Verification items for the finished model (mm, model axes). A direction names the side the tool comes from. Coordinates: 2 decimals unless noted, no trailing zeros. Order: outer loops, then holes, each group sorted by start corner. A loop starts at its lowest first (then second) coordinate and runs counter-clockwise, first axis right, second up. Notation, with made-up numbers: (16, 58) -> (64, 58) arc R7 cw to (64, 67) -> close; hole circle Ø7 at (-12, 79.5). An arc over 180 degrees is marked (long way). Write each question's results on one line, items separated by ' | '. Start each with the question number.
(1) Set-up check for faces 1 (the cylindrical face through (8.767, -16.856, 24.363)), 2 (the flat face through (-15.92, 38.95, 6.9)), 3 (the flat face through (-38.95, -15.92, 6.9)): record each of +Z, -Z, +X, -X, +Y, -Y from which the full face is reachable in a straight line by a thin tool's end or side.
(2) Cross-section at A-A on y = 2. Enter the section's corners in (x, z).
(3) Cross-section at B-B on z = 19.75. Enter the section's corners in (x, y), and give its area (3 significant figures).
(4) Cross-section at C-C on y = -14. Enter the section's corners in (x, z), and give its area (3 significant figures).
(5) Cross-section at D-D on y = 17.5. Enter the section's corners in (x, z).
(6) Draft check along Y on faces 4 (the flat face through (-41.078, -11.007, 6.902)), 5 (the flat face through (-25.46, 33.5, 6.9)), 6 (the flat face through (25.46, -33.5, 6.9)), 7 (the flat face through (-14, 27, 0)). Enter one of: +Y half, -Y half, draft (parallel to the pull), parting line (faces both ways), or undercut.
(7) Thickness scan on probe 1 along Y at (x, z) = (0, 21); probe 2 along Z at (x, y) = (36, 4.5); probe 3 along Y at (x, z) = (15, 23.75). Record the ranges inside material, lowest first. Write a range as [from, to].
(8) Go/stop test with flat-tipped pins: pin 1 (0.8 mm diameter, centred on y = 12, z = 13.5, fed in from -X); pin 2 (5 mm diameter, centred on y = 22, z = 14, fed in from +X); pin 3 (10 mm diameter, centred on x = 31.5, z = 14.5, fed in from -Y). Record where each tip stops, or that it passes through.
```python
from build123d import *

# Parameters (mm, degrees)
SKETCH1_R                  = 45
BOSS_EXTRUDE1_DEPTH        = 14
SKETCH2_R                  = 20
BOSS_EXTRUDE2_DEPTH        = 14
CUT_EXTRUDE1_DEPTH         = 70.526973183
CUT_EXTRUDE1_DEPTH_BACK    = 70.526973183
SKETCH3_R                  = 11
CUT_EXTRUDE2_DEPTH         = 70.526973183
CUT_EXTRUDE2_DEPTH_BACK    = 6
SKETCH4_R                  = 30
CUT_EXTRUDE3_DEPTH         = 70.526973183
CUT_EXTRUDE3_DEPTH_BACK    = 70.526973183
SKETCH5_W                  = 6
SKETCH5_H                  = 4.8
CUT_EXTRUDE4_DEPTH         = 70.526973183
FILLET1_R                  = 0.4
CIRPATTERN1_DEPTH          = 14
CUT_J8_CIRCLIPGROOVE_START = 23.5
SKETCH_J8_GROOVE_R         = 21.5
SKETCH_J8_GROOVE_R_2       = 19
CUT_J8_CIRCLIPGROOVE_DEPTH = 1.75


# Read off the part's stored shape, not the designer's step: CirPattern1
with BuildPart() as part:
    # Sketch1 → Boss-Extrude1 (new body)
    with BuildSketch(Plane.XY):
        Circle(SKETCH1_R)
    extrude(amount=BOSS_EXTRUDE1_DEPTH)

    # Sketch2 → Boss-Extrude2 (add)
    with BuildSketch(Plane.XY.offset(14)):
        Circle(SKETCH2_R)
    extrude(amount=BOSS_EXTRUDE2_DEPTH)

    # Sketch3 → Cut-Extrude1 (cut, two sides: drawn at the far end of the back side and taken through both)
    with BuildSketch(Plane.XY.offset(28).offset(-CUT_EXTRUDE1_DEPTH_BACK)):
        Circle(SKETCH3_R)
    extrude(amount=CUT_EXTRUDE1_DEPTH + CUT_EXTRUDE1_DEPTH_BACK, mode=Mode.SUBTRACT)

    # Sketch4 → Cut-Extrude2 (cut, two sides: drawn at the far end of the back side and taken through both)
    with BuildSketch(Plane(origin=(0, 0, 0), x_dir=(-1, 0, 0), z_dir=(0, 0, -1)).offset(-CUT_EXTRUDE2_DEPTH_BACK)):
        Circle(SKETCH4_R)
    extrude(amount=CUT_EXTRUDE2_DEPTH + CUT_EXTRUDE2_DEPTH_BACK, mode=Mode.SUBTRACT)

    # Sketch5 → Cut-Extrude3 (cut, two sides: drawn at the far end of the back side and taken through both)
    with BuildSketch(Plane.XY.offset(28).offset(-CUT_EXTRUDE3_DEPTH_BACK)):
        with Locations((0, 11)):
            Rectangle(SKETCH5_W, SKETCH5_H)
    extrude(amount=CUT_EXTRUDE3_DEPTH + CUT_EXTRUDE3_DEPTH_BACK, mode=Mode.SUBTRACT)

    # Sketch6 → Cut-Extrude4 (cut, symmetric)
    with BuildSketch(Plane(origin=(0, 0, 0), x_dir=(-1, 0, 0), z_dir=(0, 0, -1))):
        with BuildLine():
            Line((0, 40), (0, 45))
            ThreePointArc((0, 45), (-5.87367865, 44.615018762), (-11.64685703, 43.466662183))
            Line((-11.64685703, 43.466662183), (0, 40))
        make_face()
    extrude(amount=CUT_EXTRUDE4_DEPTH, both=True, mode=Mode.SUBTRACT)

    # Fillet1
    fillet1_edges = [part.edges().sort_by_distance(p)[0] for p in [
        (11.64685703, 43.466662183, 7),
    ]]
    fillet(fillet1_edges, radius=FILLET1_R)

    # CirPattern1 outline → CirPattern1 (cut)
    with BuildSketch(Plane.XY):
        with BuildLine():
            Line((10.352761804, 38.637033052), (22.386673811, 38.96802613))
            ThreePointArc((22.386673811, 38.96802613), (22.43960565, 38.965973203), (22.491802074, 38.956943945))
            Line((22.491802074, 38.956943945), (20, 34.641016151))
            Line((20, 34.641016151), (31.709533711, 31.8461253))
            ThreePointArc((31.709533711, 31.8461253), (31.760130605, 31.830442556), (31.808211535, 31.808211535))
            Line((31.808211535, 31.808211535), (28.284271247, 28.284271247))
            Line((28.284271247, 28.284271247), (38.871441292, 22.553963659))
            ThreePointArc((38.871441292, 22.553963659), (38.916255145, 22.525719852), (38.956943945, 22.491802074))
            Line((38.956943945, 22.491802074), (34.641016151, 20))
            Line((34.641016151, 20), (43.384324386, 11.724786666))
            ThreePointArc((43.384324386, 11.724786666), (43.42030121, 11.685906565), (43.450825005, 11.642613471))
            Line((43.450825005, 11.642613471), (38.637033052, 10.352761804))
            Line((38.637033052, 10.352761804), (44.94063747, 0.096584839))
            ThreePointArc((44.94063747, 0.096584839), (44.965325502, 0.049718058), (44.983604147, 0))
            Line((44.983604147, 0), (40, 0))
            Line((40, 0), (43.434320378, -11.538199086))
            ThreePointArc((43.434320378, -11.538199086), (43.44603717, -11.589858654), (43.450825005, -11.642613471))
            Line((43.450825005, -11.642613471), (38.637033052, -10.352761804))
            Line((38.637033052, -10.352761804), (38.96802613, -22.386673811))
            ThreePointArc((38.96802613, -22.386673811), (38.965973203, -22.43960565), (38.956943945, -22.491802074))
            Line((38.956943945, -22.491802074), (34.641016151, -20))
            Line((34.641016151, -20), (31.8461253, -31.709533711))
            ThreePointArc((31.8461253, -31.709533711), (31.830442556, -31.760130605), (31.808211535, -31.808211535))
            Line((31.808211535, -31.808211535), (28.284271247, -28.284271247))
            Line((28.284271247, -28.284271247), (22.553963659, -38.871441292))
            ThreePointArc((22.553963659, -38.871441292), (22.525719852, -38.916255145), (22.491802074, -38.956943945))
            Line((22.491802074, -38.956943945), (20, -34.641016151))
            Line((20, -34.641016151), (11.724786666, -43.384324386))
            ThreePointArc((11.724786666, -43.384324386), (11.685906565, -43.42030121), (11.642613471, -43.450825005))
            Line((11.642613471, -43.450825005), (10.352761804, -38.637033052))
            Line((10.352761804, -38.637033052), (0.096584839, -44.94063747))
            ThreePointArc((0.096584839, -44.94063747), (0.049718058, -44.965325502), (0, -44.983604147))
            Line((0, -44.983604147), (0, -40))
            Line((0, -40), (-11.538199086, -43.434320378))
            ThreePointArc((-11.538199086, -43.434320378), (-11.589858654, -43.44603717), (-11.642613471, -43.450825005))
            Line((-11.642613471, -43.450825005), (-10.352761804, -38.637033052))
            Line((-10.352761804, -38.637033052), (-22.386673811, -38.96802613))
            ThreePointArc((-22.386673811, -38.96802613), (-22.43960565, -38.965973203), (-22.491802074, -38.956943945))
            Line((-22.491802074, -38.956943945), (-20, -34.641016151))
            Line((-20, -34.641016151), (-31.709533711, -31.8461253))
            ThreePointArc((-31.709533711, -31.8461253), (-31.760130605, -31.830442556), (-31.808211535, -31.808211535))
            Line((-31.808211535, -31.808211535), (-28.284271247, -28.284271247))
            Line((-28.284271247, -28.284271247), (-38.871441292, -22.553963659))
            ThreePointArc((-38.871441292, -22.553963659), (-38.916255145, -22.525719852), (-38.956943945, -22.491802074))
            Line((-38.956943945, -22.491802074), (-34.641016151, -20))
            Line((-34.641016151, -20), (-43.384324386, -11.724786666))
            ThreePointArc((-43.384324386, -11.724786666), (-43.42030121, -11.685906565), (-43.450825005, -11.642613471))
            Line((-43.450825005, -11.642613471), (-38.637033052, -10.352761804))
            Line((-38.637033052, -10.352761804), (-44.94063747, -0.096584839))
            ThreePointArc((-44.94063747, -0.096584839), (-44.965325502, -0.049718058), (-44.983604147, 0))
            Line((-44.983604147, 0), (-40, 0))
            Line((-40, 0), (-43.434320378, 11.538199086))
            ThreePointArc((-43.434320378, 11.538199086), (-43.44603717, 11.589858654), (-43.450825005, 11.642613471))
            Line((-43.450825005, 11.642613471), (-38.637033052, 10.352761804))
            Line((-38.637033052, 10.352761804), (-38.96802613, 22.386673811))
            ThreePointArc((-38.96802613, 22.386673811), (-38.965973203, 22.43960565), (-38.956943945, 22.491802074))
            Line((-38.956943945, 22.491802074), (-34.641016151, 20))
            Line((-34.641016151, 20), (-31.8461253, 31.709533711))
            ThreePointArc((-31.8461253, 31.709533711), (-31.830442556, 31.760130605), (-31.808211535, 31.808211535))
            Line((-31.808211535, 31.808211535), (-28.284271247, 28.284271247))
            Line((-28.284271247, 28.284271247), (-22.553963659, 38.871441292))
            ThreePointArc((-22.553963659, 38.871441292), (-22.525719852, 38.916255145), (-22.491802074, 38.956943945))
            Line((-22.491802074, 38.956943945), (-20, 34.641016151))
            Line((-20, 34.641016151), (-11.724786666, 43.384324386))
            ThreePointArc((-11.724786666, 43.384324386), (-11.685906565, 43.42030121), (-11.642613471, 43.450825005))
            Line((-11.642613471, 43.450825005), (-10.352761804, 38.637033052))
            Line((-10.352761804, 38.637033052), (-0.096584839, 44.94063747))
            ThreePointArc((-0.096584839, 44.94063747), (-0.049718058, 44.965325502), (0, 44.983604147))
            Line((0, 44.983604147), (0, 45))
            ThreePointArc((0, 45), (-5.930124979, -44.607551129), (11.756815703, 43.437049676))
            ThreePointArc((11.756815703, 43.437049676), (11.700212353, 43.448063996), (11.642613471, 43.450825005))
            Line((11.642613471, 43.450825005), (10.352761804, 38.637033052))
        make_face()
    extrude(amount=CIRPATTERN1_DEPTH, mode=Mode.SUBTRACT)

    # Sketch_J8_Groove → Cut_J8_CirclipGroove (cut)
    with BuildSketch(Plane.XY.offset(CUT_J8_CIRCLIPGROOVE_START)):
        Circle(SKETCH_J8_GROOVE_R)
        Circle(SKETCH_J8_GROOVE_R_2, mode=Mode.SUBTRACT)
    extrude(amount=CUT_J8_CIRCLIPGROOVE_DEPTH, mode=Mode.SUBTRACT)


solid = part.part
```
Results are:
1) face 1: none | face 2: +Z, -Z, +Y | face 3: +Z, -Z, -X
2) outline: (-40.6, 0) -> (-29.93, 0) -> (-29.93, 6) -> (-10.82, 6) -> (-10.82, 28) -> (-19.9, 28) -> (-19.9, 25.25) -> (-18.89, 25.25) -> (-18.89, 23.5) -> (-19.9, 23.5) -> (-19.9, 14) -> (-40.6, 14) -> close; (10.82, 6) -> (29.93, 6) -> (29.93, 0) -> (43.77, 0) -> (43.77, 14) -> (19.9, 14) -> (19.9, 23.5) -> (18.89, 23.5) -> (18.89, 25.25) -> (19.9, 25.25) -> (19.9, 28) -> (10.82, 28) -> close
3) outline: circle Ø40 at (0, 0); hole (-3, 10.58) arc R11 ccw (long way) to (3, 10.58) -> (3, 13.4) -> (-3, 13.4) -> close | area: 861 mm2
4) outline: (-40.98, 0) -> (-26.53, 0) -> (-26.53, 6) -> (26.53, 6) -> (26.53, 0) -> (38.74, 0) -> (38.74, 14) -> (14.28, 14) -> (14.28, 23.5) -> (12.85, 23.5) -> (12.85, 25.25) -> (14.28, 25.25) -> (14.28, 28) -> (-14.28, 28) -> (-14.28, 25.25) -> (-12.85, 25.25) -> (-12.85, 23.5) -> (-14.28, 23.5) -> (-14.28, 14) -> (-40.98, 14) -> close | area: 1,190 mm2
5) outline: (-38.83, 0) -> (-24.37, 0) -> (-24.37, 6) -> (24.37, 6) -> (24.37, 0) -> (37.28, 0) -> (37.28, 14) -> (9.68, 14) -> (9.68, 23.5) -> (7.4, 23.5) -> (7.4, 25.25) -> (9.68, 25.25) -> (9.68, 28) -> (-9.68, 28) -> (-9.68, 25.25) -> (-7.4, 25.25) -> (-7.4, 23.5) -> (-9.68, 23.5) -> (-9.68, 14) -> (-38.83, 14) -> close
6) face 4: undercut | face 5: +Y half | face 6: -Y half | face 7: draft
7) probe 1: y = [-20, -11], [13.4, 20] | probe 2: z = [0, 14] | probe 3: y = [-11.66, 11.66]
8) pin 1: stops at x = -43.45 | pin 2: stops at x = 38.96 | pin 3: stops at y = -31.81
